Check sheet for the drawn part. Datum: minimum x, y, z corner. Units: mm. A direction names the side the tool comes from. Give positions to 0.01 mm unless a question says otherwise; leave off trailing zeros. Loops run counter-clockwise (first coordinate to the right, second up) from the corner with the lowest first, then second, coordinate; pieces in that order, holes last.
1. Go/stop test with flat-tipped pins: pin 1 Ø0.5 at (x, z) = (14.5, 1) entering from +Y; pin 2 Ø1.6 at (y, z) = (18.5, 3.5) entering from -X; pin 3 Ø2.5 at (x, z) = (19, 4) entering from -Y; pin 4 Ø3 at (x, y) = (28.5, 30) entering from -Z. Record where each tip stops, or that it passes through.
2. Material ranges on L1, parallel to Y at x = 17.5, z = 1.7; L2, parallel to X at y = 12.5, z = 4.5; L3, parallel to Z at x = 30.5, y = 24, recorded low to high.
3. Tool access check on the marked faces 1, 2 and 3. Record the directions out of +Z, -Z, +X, -X, +Y, -Y that give a thin tool (end or side, any length) a straight path to the whole face; none if there is none.
4. Cross-section at D-D, the plane z = 1. Record the cut outline in (x, y).
5. Cross-section at B-B, the plane y = 22. Record the cut outline in (x, z).
6. Cross-section at C-C, the plane x = 10. Record the cut outline in (y, z).
7. Cross-section at A-A, the plane z = 3.5. Record the cut outline in (x, y).
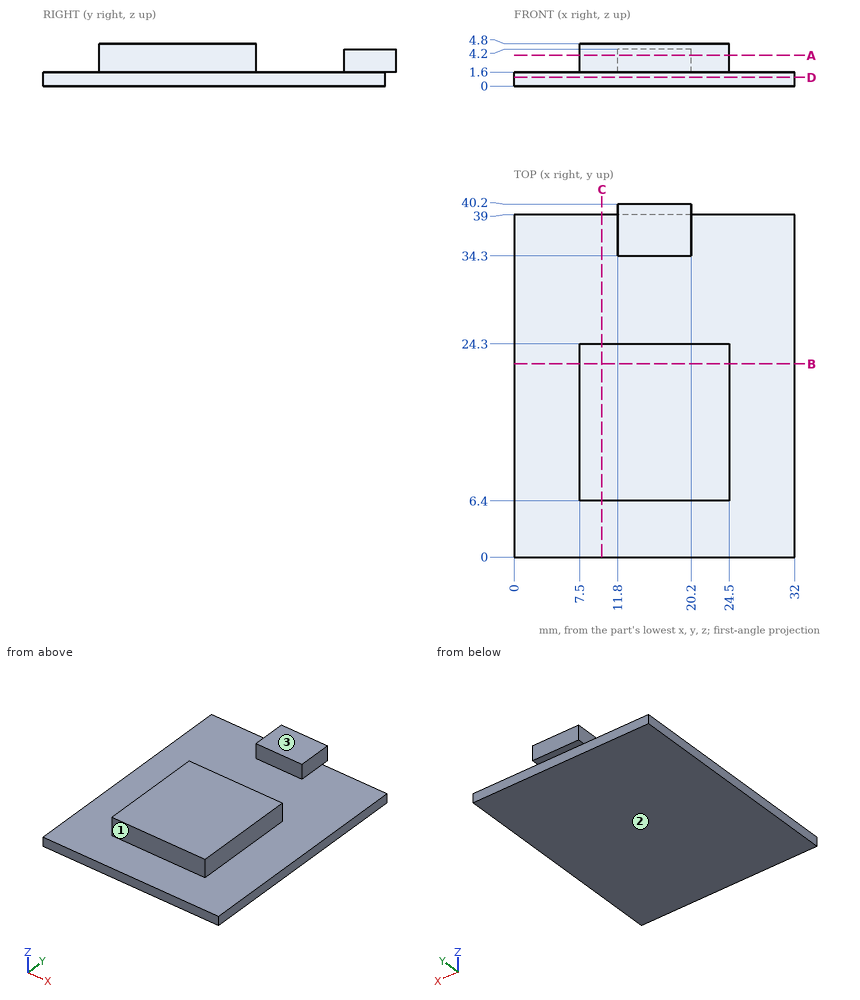
Result:
1. pin 1: stops at y = 39
1. pin 2: stops at x = 7.5
1. pin 3: stops at y = 6.4
1. pin 4: stops at z = 0
2. L1: y = 6.4 to 24.3, 34.3 to 40.2
2. L2: x = 7.5 to 24.5
2. L3: z = 0 to 1.6
3. face 1: +Z, +X, -X, -Y
3. face 2: -Z, +X, -X, +Y, -Y
3. face 3: +Z, +X, -X, +Y
4. outline: (0, 0) - (32, 0) - (32, 39) - (0, 39) - close
5. outline: (0, 0) - (32, 0) - (32, 1.6) - (24.5, 1.6) - (24.5, 4.8) - (7.5, 4.8) - (7.5, 1.6) - (0, 1.6) - close
6. outline: (0, 0) - (39, 0) - (39, 1.6) - (24.3, 1.6) - (24.3, 4.8) - (6.4, 4.8) - (6.4, 1.6) - (0, 1.6) - close
7. outline: (7.5, 6.4) - (24.5, 6.4) - (24.5, 24.3) - (7.5, 24.3) - close; (11.8, 34.3) - (20.2, 34.3) - (20.2, 40.2) - (11.8, 40.2) - close
